The listing builds one solid part. Answer for the finished solid, in the listing's coordinates (mm). Face numbers are marked on the shaded views. A direction names the side the tool comes from. Coordinates: 2 decimals unless noted, no trailing zeros. Order: outer loops, then holes, each group sorted by start corner. A loop starts at its lowest first (then second) coordinate and runs counter-clockwise, first axis right, second up. Notation, with made-up numbers: (83, 77.25) -> (101, 77.25) arc R17 ccw to (101, 90.25) -> close; hole circle Ø6 at (74, 44.5). An arc over 180 degrees is marked (long way). Answer in a Markdown table with one row per item.
```python
from build123d import *

# Parameters (mm, degrees)
F2_R     = 37.25
F3_DEPTH = 2
F5_DEPTH = 2
F6_R     = 4.99999
F7_R     = 3


# Not quite as in the source:
# - a fillet or chamfer is up to 0.001 mm smaller than in the source, because OpenCascade refuses the exact size


with BuildPart() as f1:
    # F0 (on Top) → F1 (revolve)
    with BuildSketch(Plane.XY):
        Polygon((-28.6666666667, 26.5), (-28.6666666667, 21.5), (0, 21.5), (18.6195461814, 32.25), (40.1195461814, 32.25), (40.1195461814, 37.25), (17.2798002192, 37.25), (-1.3397459622, 26.5), align=None)
    revolve(axis=Axis((-8.7595172226, 0, 0), (1, 0, 0)))

    # F2 (on face) → F3 (join)
    with BuildSketch(Plane.YZ.offset(40.1195461814)):
        Circle(F2_R)
    extrude(amount=F3_DEPTH)

    # F4 (on face) → F5 (cut, through all)
    with BuildSketch(Plane.YZ.offset(42.1195461814)):
        with BuildLine():
            ThreePointArc((32.25, 0), (31.0397930083, 8.7517855321), (27.5, 16.8467355888))
            Line((27.5, 16.8467355888), (27.5, -16.8467355888))
            ThreePointArc((27.5, -16.8467355888), (31.0397930083, -8.7517855321), (32.25, 0))
        make_face()
        with BuildLine():
            ThreePointArc((26.5, 18.3796762757), (24.1661621929, 21.3555403788), (21.5, 24.0377307581))
            Line((21.5, 24.0377307581), (21.5, -24.0377307581))
            ThreePointArc((21.5, -24.0377307581), (24.1661621929, -21.3555403788), (26.5, -18.3796762757))
            Line((26.5, -18.3796762757), (26.5, 18.3796762757))
        make_face()
        with BuildLine():
            ThreePointArc((20.5, 24.8960338207), (18.0793922843, 26.7057685647), (15.5, 28.2809564902))
            Line((15.5, 28.2809564902), (15.5, -28.2809564902))
            ThreePointArc((15.5, -28.2809564902), (18.0793922843, -26.7057685647), (20.5, -24.8960338207))
            Line((20.5, -24.8960338207), (20.5, 24.8960338207))
        make_face()
        with BuildLine():
            ThreePointArc((14.5, 28.806466288), (12.0421178111, 29.9173845552), (9.5, 30.8190282131))
            Line((9.5, 30.8190282131), (9.5, -30.8190282131))
            ThreePointArc((9.5, -30.8190282131), (12.0421178111, -29.9173845552), (14.5, -28.806466288))
            Line((14.5, -28.806466288), (14.5, 28.806466288))
        make_face()
        with BuildLine():
            ThreePointArc((8.5, 31.1096849872), (6.0187660071, 31.6833861156), (3.5, 32.0595149683))
            Line((3.5, 32.0595149683), (3.5, -32.0595149683))
            ThreePointArc((3.5, -32.0595149683), (6.0187660071, -31.6833861156), (8.5, -31.1096849872))
            Line((8.5, -31.1096849872), (8.5, 31.1096849872))
        make_face()
        with BuildLine():
            ThreePointArc((2.5, 32.1529547631), (0, 32.25), (-2.5, 32.1529547631))
            Line((-2.5, 32.1529547631), (-2.5, -32.1529547631))
            ThreePointArc((-2.5, -32.1529547631), (0, -32.25), (2.5, -32.1529547631))
            Line((2.5, -32.1529547631), (2.5, 32.1529547631))
        make_face()
        with BuildLine():
            Line((-3.5, -32.0595149683), (-3.5, 32.0595149683))
            ThreePointArc((-3.5, 32.0595149683), (-6.0187660071, 31.6833861156), (-8.5, 31.1096849872))
            Line((-8.5, 31.1096849872), (-8.5, -31.1096849872))
            ThreePointArc((-8.5, -31.1096849872), (-6.0187660071, -31.6833861156), (-3.5, -32.0595149683))
        make_face()
        with BuildLine():
            Line((-9.5, -30.8190282131), (-9.5, 30.8190282131))
            ThreePointArc((-9.5, 30.8190282131), (-12.0421178111, 29.9173845552), (-14.5, 28.806466288))
            Line((-14.5, 28.806466288), (-14.5, -28.806466288))
            ThreePointArc((-14.5, -28.806466288), (-12.0421178111, -29.9173845552), (-9.5, -30.8190282131))
        make_face()
        with BuildLine():
            Line((-15.5, -28.2809564902), (-15.5, 28.2809564902))
            ThreePointArc((-15.5, 28.2809564902), (-18.0793922843, 26.7057685647), (-20.5, 24.8960338207))
            Line((-20.5, 24.8960338207), (-20.5, -24.8960338207))
            ThreePointArc((-20.5, -24.8960338207), (-18.0793922843, -26.7057685647), (-15.5, -28.2809564902))
        make_face()
        with BuildLine():
            Line((-21.5, -24.0377307581), (-21.5, 24.0377307581))
            ThreePointArc((-21.5, 24.0377307581), (-24.1661621929, 21.3555403788), (-26.5, 18.3796762757))
            Line((-26.5, 18.3796762757), (-26.5, -18.3796762757))
            ThreePointArc((-26.5, -18.3796762757), (-24.1661621929, -21.3555403788), (-21.5, -24.0377307581))
        make_face()
        with BuildLine():
            Line((-27.5, -16.8467355888), (-27.5, 16.8467355888))
            ThreePointArc((-27.5, 16.8467355888), (-32.25, 0), (-27.5, -16.8467355888))
        make_face()
    extrude(amount=-F5_DEPTH, mode=Mode.SUBTRACT)

    # F6 (radius 5 in the source; OpenCascade refuses exactly that, so slightly less here)
    f6_edges = [f1.edges().sort_by_distance(p)[0] for p in [
        (-28.666667, -26.5, 0),
        (-1.339746, -26.5, 0),
        (17.2798, -37.25, 0),
    ]]
    fillet(f6_edges, radius=F6_R)

    # F7
    f7_edges = [f1.edges().sort_by_distance(p)[0] for p in [
        (18.619546, -32.25, 0),
        (0, -21.5, 0),
    ]]
    fillet(f7_edges, radius=F7_R)


solid = f1.part
```
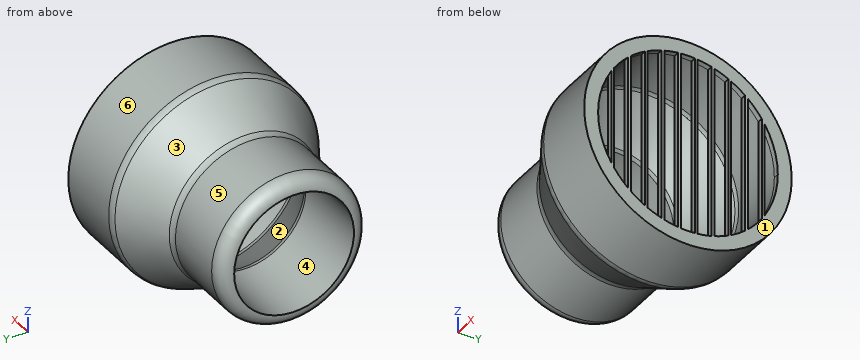
(1) A cutting plane is placed at A-A, the plane x = -14.5. Determine the outline of the cut face in (y, z).
Check values:
| item | result |
|---|---|
| outline | circle Ø53 at (0, 0); hole circle Ø43 at (0, 0) |
(2) Find the intervals of material crossed by line 1 along Y through (x, z) = (24.75, 0); line 2 along Y through (x, z) = (-14.5, 0), in increasing order. Write a range as from..to.
Check values:
| item | result |
|---|---|
| line 1 | -37.25..-32.25, 32.25..37.25 |
| line 2 | -26.5..-21.5, 21.5..26.5 |
(3) A cutting plane is placed at B-B, the plane z = -2.5. Count the separate pieces of the cut face and the enclosed holes in it, then the cut area to 3 significant figures.
Check values:
| item | result |
|---|---|
| separate pieces | 12 |
| enclosed holes | 0 |
| area | 749 mm² |
(4) Flat-ended cylindrical pins translate along their axes: pin 1 (0.5 mm diameter, centred on y = 15, z = 8.5, fed in from -X); pin 2 (2 mm diameter, centred on x = 41, z = 6, fed in from -Y); pin 3 (1.6 mm diameter, centred on x = 41, z = -3, fed in from +Y) (3 decimals); pin 4 (5 mm diameter, centred on y = 18.5, z = 8.5, fed in from -X). Find the tip coordinate at first contact, or state that the pin passes through.
Check values:
| item | result |
|---|---|
| pin 1 | x = 40.12 |
| pin 2 | y = -36.91 |
| pin 3 | y = 37.185 |
| pin 4 | x = -28.67 |
(5) Which of the six approach directions +Z, -Z, +X, -X, +Y, -Y give full straight-line access (tool end or side, diameter ignored) to the marked faces 5 and 6?
Check values:
| item | result |
|---|---|
| face 5 | -X |
| face 6 | +X, -X |
(6) For a pull along X with two mould halves and no side action, classify the marked faces 1, 2, 3 and 4 as released by +X, released by -X, zero draft, split by the parting line, or undercut.
Check values:
| item | result |
|---|---|
| face 1 | released by +X |
| face 2 | undercut |
| face 3 | released by -X |
| face 4 | zero draft |
(7) A cutting plane is placed at C-C, the plane x = 20.5. Determine the outline of the cut face in (y, z), then the cut area to 3 significant figures.
Check values:
| item | result |
|---|---|
| outline | circle Ø74.5 at (0, 0); hole circle Ø64.5 at (0, 0) |
| area | 1,090 mm² |
